Geometry check sheet. Reference: the model listing, model coordinates, mm. Face numbers are marked on the shaded views. A direction names the side the tool comes from. Round coordinates to 2 decimals unless told otherwise and drop trailing zeros. Order: outer loops, then holes, each group sorted by start corner. A loop starts at its lowest first (then second) coordinate and runs counter-clockwise, first axis right, second up.
```python
from build123d import *

# Parameters (mm, degrees)
EXTRUDE_1_DEPTH         = 23
HOLE_WIZARD_4_1_4_1_1_D = 4.1
SKETCH_5_W              = 9
SKETCH_5_H              = 13.25
CUT_EXTRUDE_1_DEPTH     = 21
EXTRUDE_2_DEPTH         = 3
HOLE_WIZARD_2_1_2_1_1_D = 2.1
SKETCH_12_W             = 3
SKETCH_12_H             = 3
EXTRUDE_4_DEPTH         = 9
FILLET_1_R              = 3


with BuildPart() as part:
    # 草图1 → 凸台-拉伸1 (new body)
    with BuildSketch(Plane(origin=(0, 0, 0), x_dir=(0, 0, -1), z_dir=(1, 0, 0))):
        Polygon((0, 0), (0, 16.25), (3, 16.25), (3, 3), (5, 3), (5, 0), align=None)
    extrude(amount=EXTRUDE_1_DEPTH)

    # Ø4.1 (4.1) 直径孔1 (through all)
    with Locations(Plane(origin=(0, 0, -3), x_dir=(-1, 0, 0), z_dir=(0, 0, -1))):
        with Locations((-4, 12.25), (-19, 12.25)):
            Hole(HOLE_WIZARD_4_1_4_1_1_D / 2)

    # 草图5 → 切除-拉伸1 (cut)
    with BuildSketch(Plane(origin=(0, 0, -3), x_dir=(-1, 0, 0), z_dir=(0, 0, -1))):
        with Locations((-11.5, 9.625)):
            Rectangle(SKETCH_5_W, SKETCH_5_H)
    extrude(amount=-CUT_EXTRUDE_1_DEPTH, mode=Mode.SUBTRACT)

    # 草图6 → 凸台-拉伸2 (add)
    with BuildSketch(Plane(origin=(0, 3, 0), x_dir=(1, 0, 0), z_dir=(0, 1, 0))):
        with BuildLine():
            ThreePointArc((3.5, 5), (1.5, 7), (-0.5, 5))
            Line((-0.5, 5), (-0.5, 0))
            Line((-0.5, 0), (0, 0))
            Line((0, 0), (0, 5))
            Line((0, 5), (3.5, 5))
        make_face()
        with BuildLine():
            Line((9.5, 0), (9.5, -2))
            ThreePointArc((9.5, -2), (11.5, -4), (13.5, -2))
            Line((13.5, -2), (13.5, 0))
            Line((13.5, 0), (9.5, 0))
        make_face()
        with BuildLine():
            Line((23.5, 0), (23.5, 5))
            ThreePointArc((23.5, 5), (21.5, 7), (19.5, 5))
            Line((19.5, 5), (23, 5))
            Line((23, 5), (23, 0))
            Line((23, 0), (23.5, 0))
        make_face()
    extrude(amount=-EXTRUDE_2_DEPTH)

    # Ø2.1 (2.1) 直径孔1 (through all)
    with Locations(Plane(origin=(0, 3, 0), x_dir=(1, 0, 0), z_dir=(0, 1, 0))):
        with Locations((1.5, 5), (11.5, -2), (21.5, 5)):
            Hole(HOLE_WIZARD_2_1_2_1_1_D / 2)

    # 草图12 → 凸台-拉伸4 (add)
    with BuildSketch(Plane.ZY.offset(-16)):
        with Locations((-1.5, 14.75)):
            Rectangle(SKETCH_12_W, SKETCH_12_H)
    extrude(amount=EXTRUDE_4_DEPTH)

    # 圆角1
    fillet_1_edges = [part.edges().sort_by_distance(p)[0] for p in [
        (23, 16.25, -1.5),
        (0, 16.25, -1.5),
    ]]
    fillet(fillet_1_edges, radius=FILLET_1_R)


solid = part.part
```
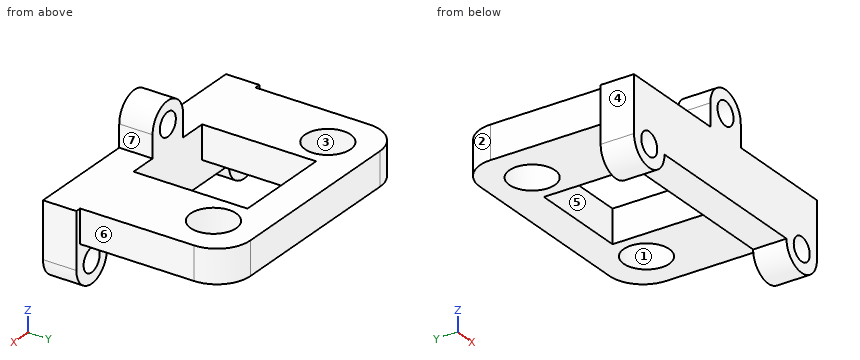
(1) Sectioned sample at B-B, the plane y = 7. Record the cut outline in (x, z), and give its area (3 significant figures).
Returned:
outline: (0, -3) - (7, -3) - (7, 0) - (0, 0) - close; (16, -3) - (23, -3) - (23, 0) - (16, 0) - close
area: 42.0 mm2
(2) Set-up check for the marked faces 5, 6 and 7: record each of +Z, -Z, +X, -X, +Y, -Y from which the full face is reachable in a straight line by a thin tool's end or side.
Returned:
face 5: +Z, -Z
face 6: +Z, -Z, +X, +Y
face 7: +Z, +X, +Y, -Y
(3) Sectioned sample at D-D, the plane x = 11.5. Record the cut outline in (y, z).
Returned:
outline: (0, -5) - (3, -5) - (3, 0.95) - (0, 0.95) - close; (0, 3.05) - (3, 3.05) - (3, 4) - (0, 4) - close; (13.25, -3) - (16.25, -3) - (16.25, 0) - (13.25, 0) - close
(4) Sectioned sample at C-C, the plane z = -2. Record the cut outline in (x, y).
Returned:
outline: (-0.5, 0) - (23.5, 0) - (23.5, 3) - (23, 3) - (23, 13.25) arc R3 ccw to (20, 16.25) - (3, 16.25) arc R3 ccw to (0, 13.25) - (0, 3) - (-0.5, 3) - close; hole circle Ø4.1 at (4, 12.25); hole (7, 3) - (16, 3) - (16, 13.25) - (7, 13.25) - close; hole circle Ø4.1 at (19, 12.25)
(5) Material ranges on line 1 (X direction, y = 14, z = -1.75); line 2 (Z direction, x = 21.5, y = 0.75); line 3 (Y direction, x = 19, z = -0.75), recorded low to high.
Returned:
line 1: x = 0.1 to 2.93, 5.07 to 17.93, 20.07 to 22.9
line 2: z = -7 to -6.05, -3.95 to 0
line 3: y = 0 to 10.2, 14.3 to 16.25
(6) Depth check by flat-ended pin: P1, Ø1.6, axis at y = 2, z = 1.5, coming from the -X side; P2, Ø6, axis at y = 8.5, z = -2.5, coming from the +X side; P3, Ø2, axis at y = 9.5, z = -5, coming from the -X side; P4, Ø6, axis at x = 12, y = 13.5, coming from the +Z side. Enter the tip coordinate at first touch or a pass-through.
Returned:
P1: stops at x = 9.5
P2: stops at x = 23
P3: passes through
P4: stops at z = 0
(7) Sectioned sample at A-A, the plane x = 19. Record the cut outline in (y, z).
Returned:
outline: (0, -5) - (3, -5) - (3, -3) - (10.2, -3) - (10.2, 0) - (0, 0) - close; (14.3, -3) - (16.25, -3) - (16.25, 0) - (14.3, 0) - close
(8) Draft check along Y on the marked faces 1, 2, 3 and 4. Enter one of: released by +Y, released by -Y, zero draft, split by the parting line, or undercut.
Returned:
face 1: undercut
face 2: released by +Y
face 3: undercut
face 4: zero draft
